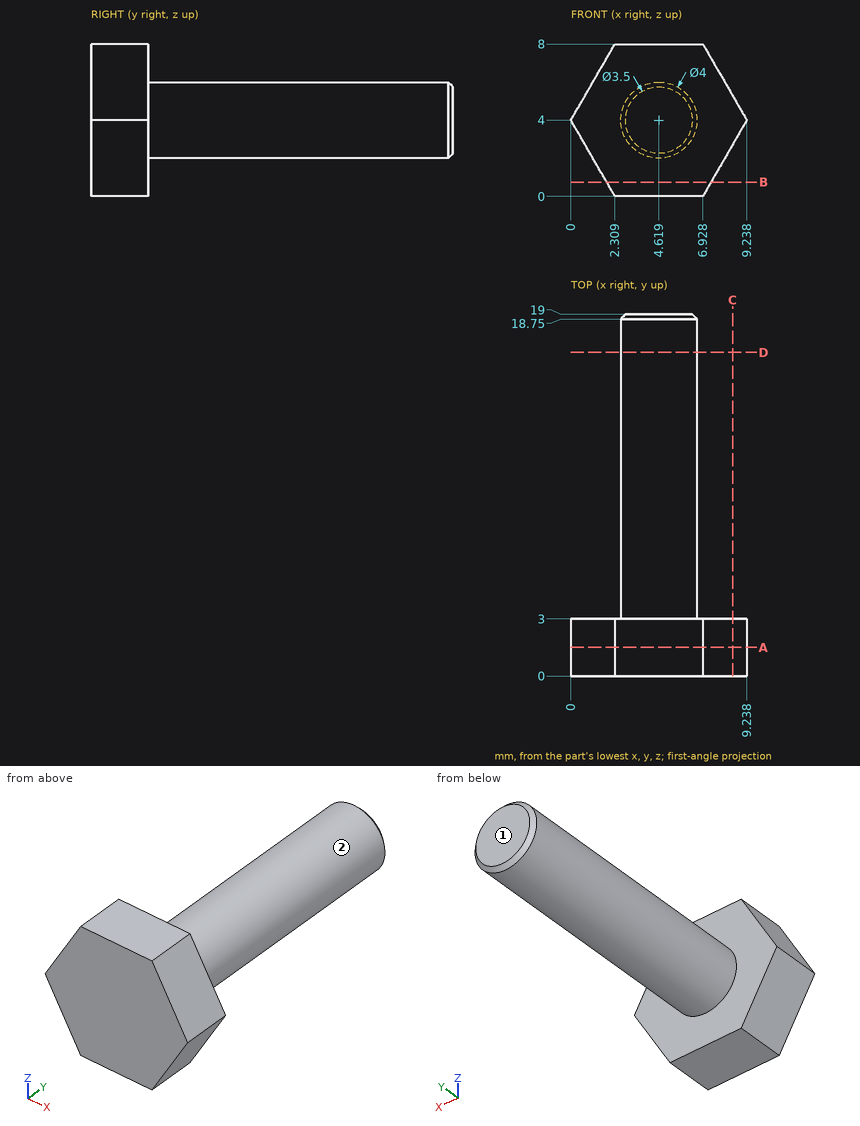
Job drawing, mm, ordinate dimensions from the low corner. One solid piece. A direction names the side the tool comes from. Coordinates: 2 decimals unless noted, no trailing zeros. Order: outer loops, then holes, each group sorted by start corner. A loop starts at its lowest first (then second) coordinate and runs counter-clockwise, first axis right, second up. Notation, with made-up numbers: (9, 83.25) -> (14, 83.25) arc R25 ccw to (14, 120.25) -> close; hole circle Ø4 at (82, 86). An arc over 180 degrees is marked (long way). Return JSON: item names as keys, results as strings. Group by question number.
Item 1: Saw through at C-C on x = 8.5. Write the cut outline in (y, z).
Item 2: Saw through at D-D on y = 17. Write the cut outline in (x, z), then the cut area to 3 significant figures.
Item 3: Wall check: line 1 along X through (y, z) = (3.75, 4); line 2 along Z through (x, y) = (4.5, 5.75); line 3 along Y through (x, z) = (4.5, 1). Give the ranges that are in metal, low to high. Write a range as [from, to].
Item 4: Saw through at A-A on y = 1.5. Write the cut outline in (x, z), then the cut area to 3 significant figures.
Item 5: Saw through at B-B on z = 0.75. Write the cut outline in (x, y).
Item 6: Flat gauge pins, fed straight in: P1, Ø1.5, axis at x = 3.5, y = 7, coming from the -Z side; P2, Ø2, axis at y = 16.5, z = 3.5, coming from the +X side; P3, Ø1.5, axis at y = 12, z = 7, coming from the +X side; P4, Ø3, axis at x = 7, y = 5, coming from the +Z side (1 decimal). Where does each tip first touch, or does it go through?
Item 7: Tool access for the marked faces 1 and 2: list every direction of +Z, -Z, +X, -X, +Y, -Y with a clear straight run to the whole face (end or side of a thin tool).
Values found:
{
 "1": {"outline": "(0, 2.72) -> (3, 2.72) -> (3, 5.28) -> (0, 5.28) -> close"},
 "2": {"outline": "circle Ø4 at (4.62, 4)", "area": "12.6 mm2"},
 "3": {"line 1": "x = [2.62, 6.62]", "line 2": "z = [2, 6]", "line 3": "y = [0, 3]"},
 "4": {"outline": "(0, 4) -> (2.31, 0) -> (6.93, 0) -> (9.24, 4) -> (6.93, 8) -> (2.31, 8) -> close", "area": "55.4 mm2"},
 "5": {"outline": "(1.88, 0) -> (7.36, 0) -> (7.36, 3) -> (1.88, 3) -> close"},
 "6": {"P1": "stops at z = 2.03", "P2": "stops at x = 6.62", "P3": "passes through", "P4": "stops at z = 5.8"},
 "7": {"face 1": "+Z, -Z, +X, -X, +Y", "face 2": "+Y"}
}
